```python
from build123d import *

# Parameters (mm, degrees)
MODEL_W                 = 52
MODEL_H                 = 52
MODEL_R                 = 1.5
SALIENTE_EXTRUIR1_DEPTH = 3


with BuildPart() as part:
    # Model → Saliente-Extruir1 (new body)
    with BuildSketch(Plane.XY):
        with Locations((26, 26)):
            Rectangle(MODEL_W, MODEL_H)
        with Locations((41, 41)):
            Circle(MODEL_R, mode=Mode.SUBTRACT)
        with Locations((41, 11)):
            Circle(MODEL_R, mode=Mode.SUBTRACT)
        with Locations((11, 11)):
            Circle(MODEL_R, mode=Mode.SUBTRACT)
        with Locations((11, 41)):
            Circle(MODEL_R, mode=Mode.SUBTRACT)
        Polygon((36, 16), (45, 16), (45, 36), (36, 36), (36, 47), (16, 47), (16, 36), (6, 36), (6, 16), (16, 16), (16, 5), (36, 5), align=None, mode=Mode.SUBTRACT)
    extrude(amount=SALIENTE_EXTRUIR1_DEPTH)


solid = part.part
```
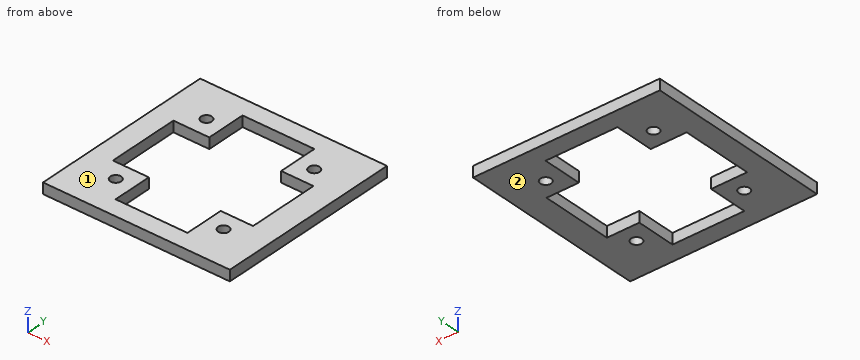
Can you work these out from the model? Positions are in its coordinate system, mm. Face numbers are marked on the shaded views. Round coordinates to 2 decimals unless told otherwise and drop trailing zeros. Loops run counter-clockwise (first coordinate to the right, second up) from the corner with the lowest first, then second, coordinate; pieces in that order, holes last. Notation, with made-up numbers: M 87.25,9.5 L 98.25,9.5 A28 ccw 98.25,38.5 Z; hole C -4.75,5 d11. An arc over 180 degrees is marked long. Answer as a JSON object with one key per item and string values. Group by question number.
Q1. Imagine slicing it at A-A, the plane y = 34. Please give me the cut outline in (x, z).
Q2. Imagine slicing it at C-C, the plane z = 0.5. Please give me the cut outline in (x, y).
Q3. Imagine slicing it at B-B, the plane x = 7.5. Please give me the cut outline in (y, z).
Q4. Imagine slicing it at D-D, the plane y = 11. Please give me the cut outline in (x, z), then the cut area to 3 significant figures.
Q5. We'd pull the mould along Z, two halves only. Please class the marked faces 1 and 2: +Z half, -Z half, draft (parallel to the pull), parting line (faces both ways), or undercut.
Q6. Please list where these lines run through material, in increasing order: L1, parallel to Y at x = 41, z = 1.5; L2, parallel to X at y = 10.5, z = 1.25; L3, parallel to Y at x = 18, z = 0.65.
Findings:
{
 "1": {"outline": "M 0,0 L 6,0 L 6,3 L 0,3 Z; M 45,0 L 52,0 L 52,3 L 45,3 Z"},
 "2": {"outline": "M 0,0 L 52,0 L 52,52 L 0,52 Z; hole M 6,16 L 16,16 L 16,5 L 36,5 L 36,16 L 45,16 L 45,36 L 36,36 L 36,47 L 16,47 L 16,36 L 6,36 Z; hole C 11,11 d3; hole C 11,41 d3; hole C 41,11 d3; hole C 41,41 d3"},
 "3": {"outline": "M 0,0 L 16,0 L 16,3 L 0,3 Z; M 36,0 L 52,0 L 52,3 L 36,3 Z"},
 "4": {"outline": "M 0,0 L 9.5,0 L 9.5,3 L 0,3 Z; M 12.5,0 L 16,0 L 16,3 L 12.5,3 Z; M 36,0 L 39.5,0 L 39.5,3 L 36,3 Z; M 42.5,0 L 52,0 L 52,3 L 42.5,3 Z", "area": "78.0 mm2"},
 "5": {"face 1": "+Z half", "face 2": "-Z half"},
 "6": {"L1": "y = 0 to 9.5, 12.5 to 16, 36 to 39.5, 42.5 to 52", "L2": "x = 0 to 9.59, 12.41 to 16, 36 to 39.59, 42.41 to 52", "L3": "y = 0 to 5, 47 to 52"}
}
